Part model, mm, in its own coordinate system. Give positions to 0.01 mm unless a question says otherwise; leave off trailing zeros. Loops run counter-clockwise (first coordinate to the right, second up) from the corner with the lowest first, then second, coordinate; pieces in that order, holes last. Notation, with made-up numbers: M 8.25,8.5 L 45.25,8.5 A29 ccw 45.25,28.5 Z; hole C 34,-8.5 d10. An arc over 180 degrees is marked long. Put each result on its own line as item: value. Start each with the question number.
```python
from build123d import *

# Parameters (mm, degrees)
SKETCH_1_W          = 50
SKETCH_1_H          = 45
EXTRUDE_1_DEPTH     = 1.5
SKETCH_2_R          = 1.6
CUT_EXTRUDE_1_DEPTH = 2
FILLET_1_R          = 2


with BuildPart() as part:
    # 草图1 → 凸台-拉伸1 (new body)
    with BuildSketch(Plane.XY):
        Rectangle(SKETCH_1_W, SKETCH_1_H)
    extrude(amount=EXTRUDE_1_DEPTH)

    # 草图2 → 切除-拉伸1 (cut)
    with BuildSketch(Plane(origin=(0, 0, 0), x_dir=(-1, 0, 0), z_dir=(0, 0, -1))):
        Polygon((18.72907323, 14.5), (-18.72907323, 14.5), (0, 0.027534323), align=None)
        Polygon((-3.27092677, -2.5), (-22, 11.972465677), (-22, -16.972465677), align=None)
        Polygon((18.72907323, -19.5), (0, -5.027534323), (-18.72907323, -19.5), align=None)
        Polygon((22, 11.972465677), (3.27092677, -2.5), (22, -16.972465677), align=None)
        with Locations((-10, 17.5)):
            Circle(SKETCH_2_R)
        with Locations((10, 17.5)):
            Circle(SKETCH_2_R)
    extrude(amount=-CUT_EXTRUDE_1_DEPTH, mode=Mode.SUBTRACT)

    # 圆角1
    fillet_1_edges = [part.edges().sort_by_distance(p)[0] for p in [
        (-3.27092677, -2.5, 0.75),
        (-22, 11.972465677, 0.75),
        (-22, -16.972465677, 0.75),
        (22, -16.972465677, 0.75),
        (22, 11.972465677, 0.75),
        (3.27092677, -2.5, 0.75),
        (18.72907323, -19.5, 0.75),
        (0, -5.027534323, 0.75),
        (-18.72907323, -19.5, 0.75),
        (0, 0.027534323, 0.75),
        (18.72907323, 14.5, 0.75),
        (-18.72907323, 14.5, 0.75),
        (25, -22.5, 0.75),
        (-25, -22.5, 0.75),
        (-25, 22.5, 0.75),
        (25, 22.5, 0.75),
    ]]
    fillet(fillet_1_edges, radius=FILLET_1_R)


solid = part.part
```
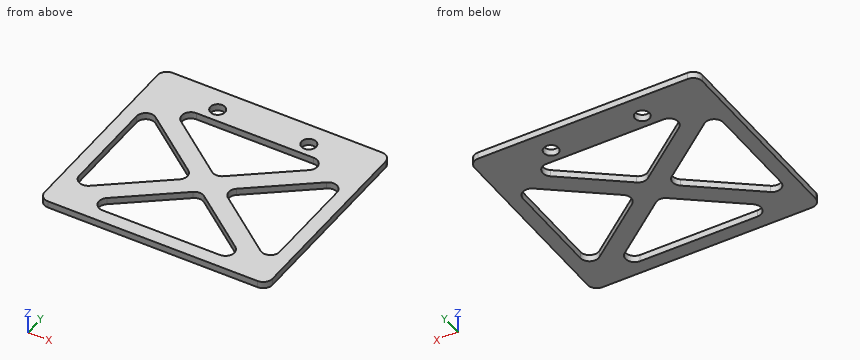
1) Band-saw the part on D-D on x = 3.5. Give the cut face in (y, z), then the cut area to 3 significant figures.
2) Wall check: L1, parallel to X at y = 8, z = 1.25; L2, parallel to X at y = -2.5, z = 1.35; L3, parallel to Y at x = 10, z = 0.8. Give the ranges that are in metal, low to high.
3) Band-saw the part on B-B on z = 1. State how many separate pieces and enclosed holes the cut face has, then the cut area to 3 significant figures.
4) Band-saw the part on C-C on x = -10. Give the cut face in (y, z).
5) Band-saw the part on A-A on y = 17.5. Give the cut face in (x, z), then the cut area to 3 significant figures.
Evaluation:
1. outline: M -22.5,0 L -19.5,0 L -19.5,1.5 L -22.5,1.5 Z; M -7.73,0 L 2.73,0 L 2.73,1.5 L -7.73,1.5 Z; M 14.5,0 L 22.5,0 L 22.5,1.5 L 14.5,1.5 Z
1. area: 32.2 mm2
2. L1: -25 to -22, -16.86 to -10.32, 10.32 to 16.86, 22 to 25
2. L2: -25 to -22, -4.54 to 4.54, 22 to 25
2. L3: -22.5 to -19.5, -12.75 to -7.7, 2.7 to 7.75, 14.5 to 15.9, 19.1 to 22.5
3. separate pieces: 1
3. enclosed holes: 6
3. area: 1,190 mm2
4. outline: M -22.5,0 L -19.5,0 L -19.5,1.5 L -22.5,1.5 Z; M -12.75,0 L -7.7,0 L -7.7,1.5 L -12.75,1.5 Z; M 2.7,0 L 7.75,0 L 7.75,1.5 L 2.7,1.5 Z; M 14.5,0 L 15.9,0 L 15.9,1.5 L 14.5,1.5 Z; M 19.1,0 L 22.5,0 L 22.5,1.5 L 19.1,1.5 Z
5. outline: M -25,0 L -11.6,0 L -11.6,1.5 L -25,1.5 Z; M -8.4,0 L 8.4,0 L 8.4,1.5 L -8.4,1.5 Z; M 11.6,0 L 25,0 L 25,1.5 L 11.6,1.5 Z
5. area: 65.4 mm2
